Autodesk Inventor part; units mm, degrees
ref_plane "YZ Plane" through (0, 0, 0) normal (1, 0, 0) x (0, 1, 0)
ref_plane "XZ Plane" through (0, 0, 0) normal (0, 1, 0) x (-1, 0, 0)
ref_plane "XY Plane" through (0, 0, 0) normal (0, 0, 1) x (1, 0, 0)
sketch "草图1" plane through (0, 0, 0) normal (0, 1, 0) x (-1, 0, 0)
  line L0 (20, -11.547) -> (0, -23.094)
  line L1 (0, -23.094) -> (-20, -11.547)
  line L2 (-20, -11.547) -> (-20, 11.547)
  line L3 (-20, 11.547) -> (0, 23.094)
  line L4 (0, 23.094) -> (20, 11.547)
  line L5 (20, 11.547) -> (20, -11.547)
  point P0 (0, 0)
  point P1 (0, 0)
  dimension "d0" = 40
extrude "拉伸1" add sketch "草图1" along normal mid plane 8
sketch "草图4" plane through (0, -4, 0) normal (0, -1, 0) x (1, 0, 0)
  circle A0 centre (0, 0) radius 18
  dimension "d18" = 36
extrude "拉伸3" add sketch "草图4" along normal blind 4
sketch "草图5" plane through (0, -8, 0) normal (0, -1, 0) x (1, 0, 0)
  circle A0 centre (0, 0) radius 20
  dimension "d21" = 40
extrude "拉伸4" add sketch "草图5" along normal blind 18
thread "螺纹1"
sketch "草图6" plane through (0, 0, 0) normal (0, 0, 1) x (1, 0, 0)
  line L0 (0, 4) -> (20, 4)
  line L1 (-20, -26) -> (20, -26)
  line L2 (0, 11.1674) -> (0, -43.9009)
  line L3 (10, -22.5359) -> (16, -26)
  line L4 (10, 4) -> (10, -22.5359)
  line L5 (20, -4) -> (20, 4)
  line L6 (0, 4) -> (20, 4)
  line L7 (0, -4) -> (0, 4)
  line L8 (20, -4) -> (0, -4)
  line L9 (-20, -26) -> (20, -26)
  line L10 (-20, -8) -> (20, -8)
  point P0 (0, 0)
  point P1 (0, -26)
  dimension "d28" = 60
  dimension "d29" = 16
revolve "旋转2" cut sketch "草图6" angle 360 about axis through (0, 11.1674, 0) along (0, -1, 0) contours L0 L4 L8 L2 | L8 L4 L10 L2 | L10 L4 L3 L1 L2
chamfer "倒角2" distance 1.5 angle 45 1 edges at (-20, -26, 0)
properties part number "螺套" material "不锈钢"
Geometry check sheet. Reference: the model listing, model coordinates, mm. A direction names the side the tool comes from. Give positions to 0.01 mm unless a question says otherwise; leave off trailing zeros. Order: outer loops, then holes, each group sorted by start corner. A loop starts at its lowest first (then second) coordinate and runs counter-clockwise, first axis right, second up. Notation, with made-up numbers: (0, -26.75) - (16, -26.75) arc R10 ccw to (16, -11.75) - close; hole circle Ø4 at (84, 4.5). An arc over 180 degrees is marked (long way). Answer in a Markdown table with one row per item. Add a question column.
Q1. Cross-section at C-C, the plane y = -11. Enter the section's corners in (x, z), then the cut area to 3 significant figures.
Q2. Tool access check on faces 4 (the flat face through (20, 0, 0)), 5 (the flat face through (12, -4, -14)), 6 (the cylindrical face through (-4.336, -16.134, 19.524)). Record the directions out of +Z, -Z, +X, -X, +Y, -Y that give a thin tool (end or side, any length) a straight path to the whole face; none if there is none.
Q3. Cross-section at B-B, the plane z = 0. Enter the section's corners in (x, y), then the cut area to 3 significant figures.
Q4. Mould release check, pull along Y, two halves, no side actions. Record for faces 1 (the flat face through (9.86, -0.06, -17.4)), 2 (the flat face through (9, 4, -5)), 3 (the flat face through (-18, -8, 3)): pulls with the +Y half, pulls with the -Y half, needs draft (parallel to the pull), parting line crosses it, or undercut.
Q5. Material ranges on probe 1 along Z at (x, y) = (0, -14); probe 2 along X at (y, z) = (-14.25, -7) (3 decimals); probe 3 along Y at (x, z) = (-9.5, 16), recorded low to high. Write a range as from..to.
Q6. Cross-section at A-A, the plane y = -2. Enter the section's corners in (x, z), then the cut area to 3 significant figures.
Q7. Gauge pin test, flat ends, axial feed: pin 1 (3 mm diameter, centred on x = 9, z = -10.5, fed in from -Y); pin 2 (12 mm diameter, centred on x = -0.5, z = 4, fed in from -Y); pin 3 (3 mm diameter, centred on x = -12, z = 1.5, fed in from -Y). Record the tip position at first contact, or that the pin passes through.
Check values:
| question | item | result |
|---|---|---|
| 1 | outline | circle Ø40 at (0, 0); hole circle Ø20 at (0, 0) |
| 1 | area | 942 mm^2 |
| 2 | face 4 | +Z, -Z, +X, +Y, -Y |
| 2 | face 5 | none |
| 2 | face 6 | -Y |
| 3 | outline | (-20, -24.5) - (-18.5, -26) - (-16, -26) - (-10, -22.54) - (-10, 4) - (-20, 4) - (-20, -4) - (-18, -4) - (-18, -8) - (-20, -8) - close; (10, -22.54) - (16, -26) - (18.5, -26) - (20, -24.5) - (20, -8) - (18, -8) - (18, -4) - (20, -4) - (20, 4) - (10, 4) - close |
| 3 | area | 561 mm^2 |
| 4 | face 1 | needs draft |
| 4 | face 2 | pulls with the +Y half |
| 4 | face 3 | undercut |
| 5 | probe 1 | z = -20..-10, 10..20 |
| 5 | probe 2 | x = -18.735..-7.141, 7.141..18.735 |
| 5 | probe 3 | y = -25.89..-8, -4..4 |
| 6 | outline | (-20, -11.55) - (0, -23.09) - (20, -11.55) - (20, 11.55) - (0, 23.09) - (-20, 11.55) - close; hole circle Ø20 at (0, 0) |
| 6 | area | 1,070 mm^2 |
| 7 | pin 1 | stops at y = -25.61 |
| 7 | pin 2 | stops at y = -22.55 |
| 7 | pin 3 | stops at y = -24.61 |
